Job drawing, mm, ordinate dimensions from the low corner. One solid piece. A direction names the side the tool comes from. Round coordinates to 2 decimals unless told otherwise and drop trailing zeros. Loops run counter-clockwise (first coordinate to the right, second up) from the corner with the lowest first, then second, coordinate; pieces in that order, holes last. Notation, with made-up numbers: (11, -30.75) - (32, -30.75) arc R20 cw to (32, -8.75) - close; hole circle Ø9 at (-31, -8.5). An arc over 180 degrees is marked (long way). Answer as CSV lines item,"result". Start each with the question number.
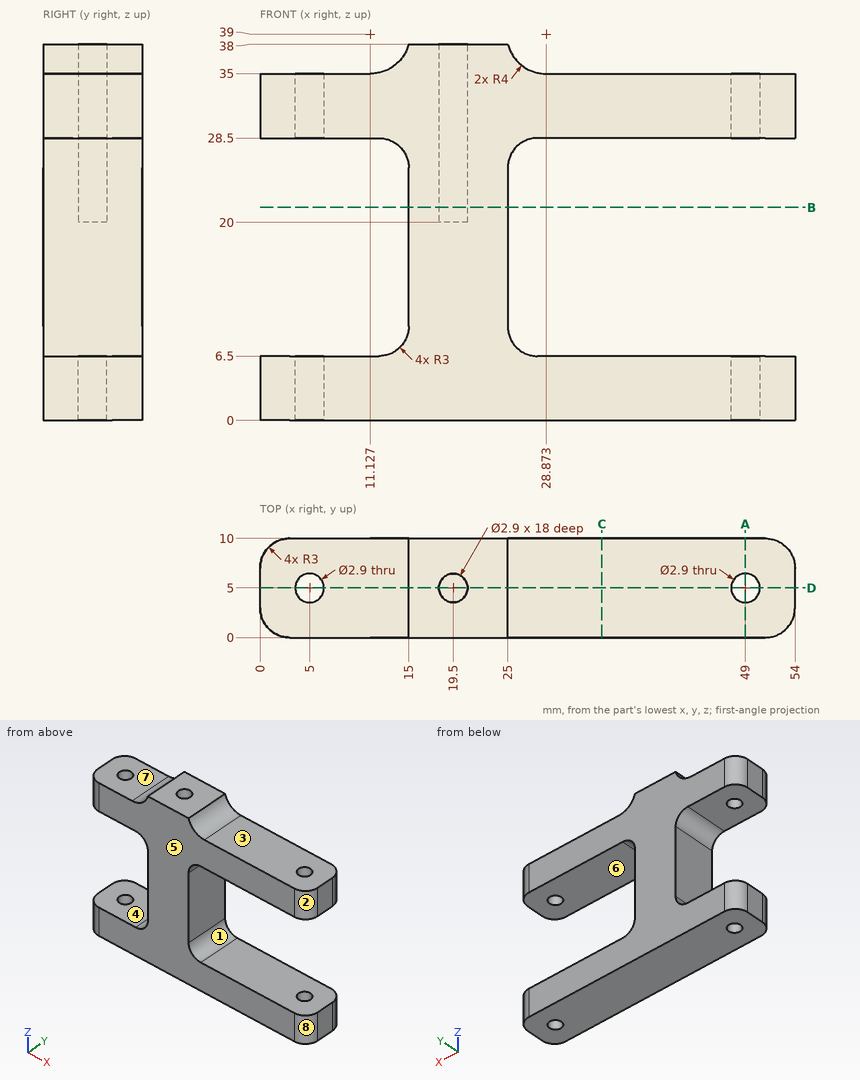
Q1. Band-saw the part on D-D, the plane y = 5. Give the number of separate pieces and of enclosed holes in the cut face, then the cut area to 3 significant figures.
Q2. Two-plate mould, pull along Z, no slides. Class the marked faces 1, 2 and 3: released by +Z, released by -Z, zero draft, split by the parting line, or undercut.
Q3. Wall check: probe 1 along Z at (x, y) = (37, 8.75); probe 2 along Y at (x, z) = (49, 2); probe 3 along X at (y, z) = (4.5, 3.5). Give the ranges that are in metal, low to high. Write a range as [from, to].
Q4. Band-saw the part on B-B, the plane z = 21.5. List the corners of the cut face in (x, y).
Q5. Tool access for the marked faces 4, 5, 6, 7 and 8: list every direction of +Z, -Z, +X, -X, +Y, -Y with a clear straight run to the whole face (end or side of a thin tool).
Q6. Pin check, flat tips, straight feed: pin 1 Ø0.9 at (x, y) = (19.5, 4.5) entering from +Z; pin 2 Ø5 at (x, y) = (37.5, 5) entering from +Z; pin 3 Ø2 at (y, z) = (6, 26) entering from +X. Stop position of each tip, or through.
Q7. Band-saw the part on C-C, the plane x = 34.5. List the corners of the cut face in (y, z), then the cut area to 3 significant figures.
Q8. Band-saw the part on A-A, the plane x = 49. List the corners of the cut face in (y, z).
Reported:
1,separate pieces,"5"
1,enclosed holes,"0"
1,area,"838 mm2"
2,face 1,"undercut"
2,face 2,"zero draft"
2,face 3,"released by +Z"
3,probe 1,"z = [0, 6.5], [28.5, 35]"
3,probe 2,"y = [0, 3.55], [6.45, 10]"
3,probe 3,"x = [0, 3.64], [6.36, 47.64], [50.36, 54]"
4,outline,"(15, 0) - (25, 0) - (25, 10) - (15, 10) - close; hole circle Ø2.9 at (19.5, 5)"
5,face 4,"-X, +Y, -Y"
5,face 5,"+Z, -Z, +X, -X, -Y"
5,face 6,"+X, +Y, -Y"
5,face 7,"+Z, -X, +Y, -Y"
5,face 8,"+Z, -Z, +X, -Y"
6,pin 1,"stops at z = 20"
6,pin 2,"stops at z = 35"
6,pin 3,"stops at x = 25.4"
7,outline,"(0, 0) - (10, 0) - (10, 6.5) - (0, 6.5) - close; (0, 28.5) - (10, 28.5) - (10, 35) - (0, 35) - close"
7,area,"130 mm2"
8,outline,"(0, 0) - (3.55, 0) - (3.55, 6.5) - (0, 6.5) - close; (0, 28.5) - (3.55, 28.5) - (3.55, 35) - (0, 35) - close; (6.45, 0) - (10, 0) - (10, 6.5) - (6.45, 6.5) - close; (6.45, 28.5) - (10, 28.5) - (10, 35) - (6.45, 35) - close"
